The model under review builds one solid part; all positions refer to its coordinate system, in mm. A direction names the side the tool comes from. Round coordinates to 2 decimals unless told otherwise and drop trailing zeros. Loops run counter-clockwise (first coordinate to the right, second up) from the corner with the lowest first, then second, coordinate; pieces in that order, holes last. Notation, with made-up numbers: (-33, 7) -> (-17, 7) arc R30 ccw to (-17, 45) -> close; hole circle Ø8 at (25.25, 55). An arc over 180 degrees is marked (long way). Return JSON: item names as keys, results as strings. Group by question number.
Autodesk Inventor part; units mm, degrees
ref_plane "Work Plane1" through (3.5, 0, 0) normal (1, 0, 0) x (0, 1, 0)
ref_plane "XZ Plane" through (0, 0, 0) normal (0, 1, 0) x (-1, 0, 0)
ref_plane "XY Plane" through (0, 0, 0) normal (0, 0, 1) x (1, 0, 0)
sketch "Sketch1" plane through (0, 0, 0) normal (0, 0, 1) x (1, 0, 0)
  line L0 (0, 0) -> (0, 6)
  line L1 (0, 6) -> (7, 6)
  line L2 (7, 6) -> (7, 0)
  line L3 (7, 0) -> (0, 0)
  dimension "d0" = 12
  dimension "d1" = 7
revolve "Revolution1" add sketch "Sketch1" angle 360 about axis through (7, 0, 0) along (-1, 0, 0)
ref_plane "Work Plane1" through (3.5, 0, 0) normal (1, 0, 0) x (0, 1, 0)
sketch "Sketch2" plane through (3.5, 0, 0) normal (1, 0, 0) x (0, 1, 0)
  line L0 (-2.5, 2.5) -> (2.5, 2.5)
  line L1 (2.5, 2.5) -> (2.5, -2.5)
  line L2 (2.5, -2.5) -> (-2.5, -2.5)
  line L3 (-2.5, -2.5) -> (-2.5, 2.5)
  line L4 (-2.5, 2.5) -> (2.5, -2.5) construction
  line L5 (2.5, 2.5) -> (-2.5, -2.5) construction
  point P0 (0, 0)
  dimension "d3" = 5
  dimension "d4" = 5
extrude "Extrusion1" add sketch "Sketch2" along normal mid plane 17
properties part number "210 part 3"
1. We need section C-C, the plane x = 6.5. Write out the cut boundary in (y, z).
2. We need section D-D, the plane z = 4.75. Write out the cut boundary in (x, y).
3. We need section A-A, the plane y = -0.75. Write out the cut boundary in (x, z), then the cut area to 3 significant figures.
4. Tool access review of faces 1 (the face through (-3, 2.5, 0)), 2 (the face through (9, 0, 2.5)), 3 (the face through (-3, 0, 2.5)): name each direction out of +Z, -Z, +X, -X, +Y, -Y from which nothing blocks a thin tool from reaching the whole face with its end or side.
5. We need section B-B, the plane z = 0. Write out the cut boundary in (x, y), then the cut area to 3 significant figures.
6. Wall thickness on line 1 (X direction, y = -4.5, z = 2.25); line 2 (Z direction, x = -2.25, y = 2); line 3 (Z direction, x = 3, y = -3): over which ranges is each line inside the solid? List them lowest first.
7. For P1, Ø4, axis at x = 10, y = -0.5, coming from the -Z side; P2, Ø1.5, axis at x = -1.5, z = -1, coming from the -Y side; P3, Ø5.5, axis at x = -3.5, z = 1, coming from the +Y side, all flat-tipped, find the tip position at first contact; note any pin that passes through.
Check sheet entries:
{
 "1": {"outline": "circle Ø12 at (0, 0)"},
 "2": {"outline": "(0, -3.67) -> (7, -3.67) -> (7, 3.67) -> (0, 3.67) -> close"},
 "3": {"outline": "(-5, -2.5) -> (0, -2.5) -> (0, -5.95) -> (7, -5.95) -> (7, -2.5) -> (12, -2.5) -> (12, 2.5) -> (7, 2.5) -> (7, 5.95) -> (0, 5.95) -> (0, 2.5) -> (-5, 2.5) -> close", "area": "133 mm²"},
 "4": {"face 1": "+Z, -Z, -X, +Y", "face 2": "+Z, +X, +Y, -Y", "face 3": "+Z, -X, +Y, -Y"},
 "5": {"outline": "(-5, -2.5) -> (0, -2.5) -> (0, -6) -> (7, -6) -> (7, -2.5) -> (12, -2.5) -> (12, 2.5) -> (7, 2.5) -> (7, 6) -> (0, 6) -> (0, 2.5) -> (-5, 2.5) -> close", "area": "134 mm²"},
 "6": {"line 1": "x = 0 to 7", "line 2": "z = -2.5 to 2.5", "line 3": "z = -5.2 to 5.2"},
 "7": {"P1": "stops at z = -2.5", "P2": "stops at y = -2.5", "P3": "stops at y = 2.5"}
}
